CAD build for the part. Positions are in the model's coordinates, mm. Face numbers are marked on the shaded views. A direction names the side the tool comes from. Coordinates: 2 decimals unless noted, no trailing zeros. Loops run counter-clockwise (first coordinate to the right, second up) from the corner with the lowest first, then second, coordinate; pieces in that order, holes last. Notation, with made-up numbers: (-1, -34) -> (49, -34) arc R10 ccw to (49, -28) -> close; hole circle Ø7 at (84, 37). An arc over 180 degrees is marked (long way). Answer as CSV lines item,"result". Start each with the question number.
```python
from build123d import *

# Parameters (mm, degrees)
SKETCH1_W                    = 12.1
SKETCH1_H                    = 10.8
BASE_DEPTH                   = 8
CONTACT_OPENING_DEPTH        = 9
CONTACT_OPENING_LEAD_IN_SIZE = 0.5
SKETCH3_W                    = 5.6
SKETCH3_H                    = 3.18
CONTACT_AREA_DEPTH           = 8.5
CONTACT_AREA_LEAD_IN_SIZE    = 0.5
GROUND_LEGS_DEPTH            = 2.52
GROUND_LEGS_SHAPE_DEPTH      = 0.3
SM_TAILS_DEPTH               = 0.3
CONTACT_DEPTH                = 0.375
CONTACT_PATTERN_COUNT        = 2
CONTACT_PATTERN_PITCH        = 2.5
LPATTERN1_COUNT              = 2
LPATTERN1_PITCH              = 1.25
LPATTERN1_COL_COUNT          = 3
LPATTERN1_COL_PITCH          = 1.25
SKETCH12_R                   = 0.575
ALIGNMENT_PIN_DEPTH          = 1.9
PIN_POINT_SIZE               = 0.05


with BuildPart() as part:
    # Sketch1 → Base (new body, symmetric)
    with BuildSketch(Plane.XY):
        Rectangle(SKETCH1_W, SKETCH1_H)
    extrude(amount=BASE_DEPTH, both=True)

    # Sketch2 → Contact Opening (cut)
    with BuildSketch(Plane.XY.offset(8)):
        with BuildLine():
            Line((-2.975, 3.94), (-4.225, 2.69))
            Line((-4.225, 2.69), (-4.225, -3.34))
            ThreePointArc((-4.225, -3.34), (-4.078553391, -3.693553391), (-3.725, -3.84))
            Line((-3.725, -3.84), (3.725, -3.84))
            ThreePointArc((3.725, -3.84), (4.078553391, -3.693553391), (4.225, -3.34))
            Line((4.225, -3.34), (4.225, 2.69))
            Line((4.225, 2.69), (2.975, 3.94))
            Line((2.975, 3.94), (-2.975, 3.94))
        make_face()
    extrude(amount=-CONTACT_OPENING_DEPTH, mode=Mode.SUBTRACT)

    # Contact Opening Lead-in
    contact_opening_lead_in_edges = [part.edges().sort_by_distance(p)[0] for p in [
        (0, 3.94, 8),
        (-3.6, 3.315, 8),
        (-4.225, -0.325, 8),
        (-4.078553391, -3.693553391, 8),
        (0, -3.84, 8),
        (4.078553391, -3.693553391, 8),
        (4.225, -0.325, 8),
        (3.6, 3.315, 8),
    ]]
    chamfer(contact_opening_lead_in_edges, length=CONTACT_OPENING_LEAD_IN_SIZE)

    # Sketch3 → Contact Area (add)
    with BuildSketch(Plane.XY.offset(-1)):
        with Locations((0, 0.05)):
            Rectangle(SKETCH3_W, SKETCH3_H)
    extrude(amount=CONTACT_AREA_DEPTH)

    # Contact Area Lead-in
    contact_area_lead_in_edges = [part.edges().sort_by_distance(p)[0] for p in [
        (-2.8, 0.05, 7.5),
        (0, -1.54, 7.5),
        (2.8, 0.05, 7.5),
        (0, 1.64, 7.5),
    ]]
    chamfer(contact_area_lead_in_edges, length=CONTACT_AREA_LEAD_IN_SIZE)

    # Sketch4 → Ground Legs (add, symmetric)
    with BuildSketch(Plane.XY.offset(-1.58)):
        with BuildLine():
            Line((6.02, -5.058034034), (5.72, -5.100661668))
            ThreePointArc((5.72, -5.100661668), (5.776842077, -5.318050295), (5.90868722, -5.5))
            Line((5.90868722, -5.5), (8.1, -5.5))
            Line((8.1, -5.5), (8.1, -5.2))
            Line((8.1, -5.2), (6.599504335, -5.2))
            ThreePointArc((6.599504335, -5.2), (6.254059507, -5.356354169), (6.02, -5.058034034))
        make_face()
        with BuildLine():
            Line((-5.90868722, -5.5), (-8.1, -5.5))
            Line((-8.1, -5.5), (-8.1, -5.2))
            Line((-8.1, -5.2), (-6.599504335, -5.2))
            ThreePointArc((-6.599504335, -5.2), (-6.254059507, -5.356354169), (-6.02, -5.058034034))
            Line((-6.02, -5.058034034), (-5.72, -5.100661668))
            ThreePointArc((-5.72, -5.100661668), (-5.776842077, -5.318050295), (-5.90868722, -5.5))
        make_face()
    extrude(amount=GROUND_LEGS_DEPTH, both=True)

    # Sketch9 → ground legs shape (cut)
    with BuildSketch(Plane(origin=(0, -5.2, 0), x_dir=(-1, 0, 0), z_dir=(0, 1, 0))):
        with BuildLine():
            Line((-8.1, -4.1), (-8.1, -3.6))
            ThreePointArc((-8.1, -3.6), (-7.953553391, -3.953553391), (-7.6, -4.1))
            Line((-7.6, -4.1), (-8.1, -4.1))
        make_face()
        Polygon((-8.1, -2.875946044), (-6.946732983, -2.33830257), (-6.946732983, -0.82169743), (-8.1, -0.284053956), align=None)
        with BuildLine():
            Line((-8.1, 0.94), (-7.6, 0.94))
            ThreePointArc((-7.6, 0.94), (-7.953553391, 0.793553391), (-8.1, 0.44))
            Line((-8.1, 0.44), (-8.1, 0.94))
        make_face()
        with BuildLine():
            Line((8.1, 0.94), (8.1, 0.44))
            ThreePointArc((8.1, 0.44), (7.953553391, 0.793553391), (7.6, 0.94))
            Line((7.6, 0.94), (8.1, 0.94))
        make_face()
        Polygon((8.1, -0.284053956), (6.946732983, -0.82169743), (6.946732983, -2.33830257), (8.1, -2.875946044), align=None)
        with BuildLine():
            Line((8.1, -4.1), (7.6, -4.1))
            ThreePointArc((7.6, -4.1), (7.953553391, -3.953553391), (8.1, -3.6))
            Line((8.1, -3.6), (8.1, -4.1))
        make_face()
    extrude(amount=-GROUND_LEGS_SHAPE_DEPTH, mode=Mode.SUBTRACT)

    # Sketch11 → SM Tails (add, symmetric)
    with BuildSketch(Plane(origin=(0.75, 0, 0), x_dir=(0, 0, -1), z_dir=(1, 0, 0))):
        with BuildLine():
            Line((7.15, -5.3), (7.15, -5.15))
            Line((7.15, -5.15), (7.4, -5.15))
            ThreePointArc((7.4, -5.15), (7.429289322, -5.220710678), (7.5, -5.25))
            Line((7.5, -5.25), (9.15, -5.25))
            Line((9.15, -5.25), (9.15, -5.5))
            Line((9.15, -5.5), (7.35, -5.5))
            ThreePointArc((7.35, -5.5), (7.208578644, -5.441421356), (7.15, -5.3))
        make_face()
    sm_tails = extrude(amount=SM_TAILS_DEPTH, both=True)

    # Sketch8 → Contact (add, symmetric)
    with BuildSketch(Plane(origin=(-1.25, 0, 0), x_dir=(0, 0, -1), z_dir=(1, 0, 0))):
        with BuildLine():
            Line((1, 1.64), (-2.511141434, 2.21990157))
            ThreePointArc((-2.511141434, 2.21990157), (-3.280012008, 2.246903627), (-4.030467404, 2.077469952))
            Line((-4.030467404, 2.077469952), (-5.5, 1.54))
            Line((-5.5, 1.54), (-5.439889401, 1.375647586))
            Line((-5.439889401, 1.375647586), (-3.970356805, 1.913117538))
            ThreePointArc((-3.970356805, 1.913117538), (-3.263677974, 2.072667582), (-2.539658184, 2.047240645))
            Line((-2.539658184, 2.047240645), (0.97148325, 1.467339075))
            Line((0.97148325, 1.467339075), (1, 1.64))
        make_face()
        with BuildLine():
            Line((-5.439889401, -1.275647586), (-5.5, -1.44))
            Line((-5.5, -1.44), (-4.030467404, -1.977469952))
            ThreePointArc((-4.030467404, -1.977469952), (-3.280012008, -2.146903627), (-2.511141434, -2.11990157))
            Line((-2.511141434, -2.11990157), (1, -1.54))
            Line((1, -1.54), (0.97148325, -1.367339075))
            Line((0.97148325, -1.367339075), (-2.539658184, -1.947240645))
            ThreePointArc((-2.539658184, -1.947240645), (-3.263677974, -1.972667582), (-3.970356805, -1.813117538))
            Line((-3.970356805, -1.813117538), (-5.439889401, -1.275647586))
        make_face()
    contact = extrude(amount=CONTACT_DEPTH, both=True)

    # Contact Pattern: Contact ×2
    with Locations(*[(i * CONTACT_PATTERN_PITCH, 0, 0) for i in range(1, CONTACT_PATTERN_COUNT)]):
        add(contact)

    # LPattern1: SM Tails ×2
    with Locations(*[(i * LPATTERN1_PITCH, 0, 0) for i in range(1, LPATTERN1_COUNT)]):
        add(sm_tails)

    # LPattern1 col: SM Tails ×3
    with Locations(*[(-i * LPATTERN1_COL_PITCH, 0, 0) for i in range(1, LPATTERN1_COL_COUNT)]):
        add(sm_tails)

    # Sketch12 → Alignment Pin (add)
    with BuildSketch(Plane.XZ.offset(5.4)):
        with Locations((2.75, -1)):
            Circle(SKETCH12_R)
        with Locations((-2.75, -1)):
            Circle(SKETCH12_R)
    extrude(amount=ALIGNMENT_PIN_DEPTH)

    # Pin Point
    pin_point_edges = [part.edges().sort_by_distance(p)[0] for p in [
        (2.175, -7.3, -1),
        (-3.325, -7.3, -1),
    ]]
    chamfer(pin_point_edges, length=PIN_POINT_SIZE)


solid = part.part
```
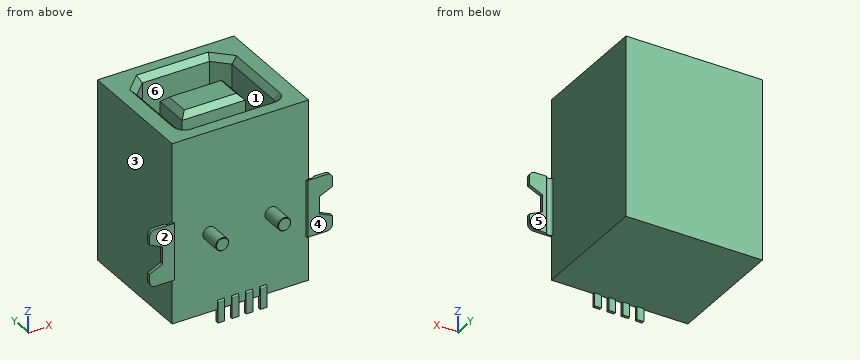
Q1. Which spindle directions (+Z, -Z, +X, -X, +Y, -Y) get a long thin tool onto all of the face, cutting with end or side? Do the marked faces 4, 5 and 6. Say none if no direction does.
Q2. Saw through at A-A (y = -0.25). List the corners of the cut face in (x, z) (3 decimals), and give its area (3 significant figures).
Q3. Probe probe 1 along X at (y, z) = (1.75, 4.5) (3 decimals); probe 2 along X at (y, z) = (1.5, 4.5) (3 decimals); probe 3 along Y at (x, z) = (-2.75, 2). List the from-to ranges inside material, lowest first. Write a range as from..to.
Q4. Saw through at B-B (y = -6). List the corners of the cut face in (x, z) (3 decimals).
Q5. Pin check, flat tips, straight feed: pin 1 Ø1.6 at (y, z) = (0, 4.5) entering from -X; pin 2 Ø1.8 at (y, z) = (-0.5, 5) entering from +X; pin 3 Ø5 at (x, z) = (1, 2) entering from -Y. Stop position of each tip, or through.
Q6. Two-plate mould, pull along X, no slides. Class the marked faces 1, 2 and 3: pulls with the +X half, pulls with the -X half, needs draft (parallel to the pull), parting line crosses it, or undercut.
Q7. Saw through at C-C (x = -5). List the corners of the cut face in (y, z), and give its area (3 significant figures).
Ans:
1,face 4,"+Z, -Z, +X, -Y"
1,face 5,"+Z, -Z, +X, +Y"
1,face 6,"+Z"
2,outline,"(-6.05, -8) -> (6.05, -8) -> (6.05, 8) -> (4.725, 8) -> (4.225, 7.5) -> (4.225, -1) -> (2.8, -1) -> (2.8, 7) -> (2.3, 7.5) -> (-2.3, 7.5) -> (-2.8, 7) -> (-2.8, -1) -> (-4.225, -1) -> (-4.225, 7.5) -> (-4.725, 8) -> (-6.05, 8) -> close"
2,area,"165 mm²"
3,probe 1,"x = -6.05..-4.225, -1.625..-0.875, 0.875..1.625, 4.225..6.05"
3,probe 2,"x = -6.05..-4.225, -2.8..2.8, 4.225..6.05"
3,probe 3,"y = -5.4..-3.84, -1.54..1.64, 3.94..5.4"
4,outline,"circle Ø1.15 at (-2.75, -1); circle Ø1.15 at (2.75, -1)"
5,pin 1,"stops at x = -6.05"
5,pin 2,"stops at x = 6.05"
5,pin 3,"stops at y = -5.4"
6,face 1,"undercut"
6,face 2,"needs draft"
6,face 3,"pulls with the -X half"
7,outline,"(-5.4, -8) -> (5.4, -8) -> (5.4, 8) -> (-5.4, 8) -> close"
7,area,"173 mm²"
